from build123d import *

# Parameters (mm, degrees)
ESBO_O1_R                = 1.25
ESBO_O1_R_2              = 0.5
RESSALTO_EXTRUS_O1_DEPTH = 2
ESBO_O2_R                = 3.25
ESBO_O2_R_2              = 2.1
RESSALTO_EXTRUS_O2_DEPTH = 2.2


with BuildPart() as part:
    # Esboço1 → Ressalto-extrusão1 (new body)
    with BuildSketch(Plane.XY):
        with BuildLine():
            Line((16.1640625, 1.742292598), (0.3046875, 3.235686253))
            ThreePointArc((0.3046875, 3.235686253), (-3.25, 0), (0.3046875, -3.235686253))
            Line((0.3046875, -3.235686253), (16.1640625, -1.742292598))
            ThreePointArc((16.1640625, -1.742292598), (17.75, 0), (16.1640625, 1.742292598))
        make_face()
        Circle(ESBO_O1_R, mode=Mode.SUBTRACT)
        with Locations((16, 0)):
            Circle(ESBO_O1_R_2, mode=Mode.SUBTRACT)
        with Locations((14.03, 0)):
            Circle(ESBO_O1_R_2, mode=Mode.SUBTRACT)
        with Locations((12.06, 0)):
            Circle(ESBO_O1_R_2, mode=Mode.SUBTRACT)
        with Locations((10.09, 0)):
            Circle(ESBO_O1_R_2, mode=Mode.SUBTRACT)
        with Locations((8.12, 0)):
            Circle(ESBO_O1_R_2, mode=Mode.SUBTRACT)
        with Locations((6.15, 0)):
            Circle(ESBO_O1_R_2, mode=Mode.SUBTRACT)
        with Locations((4.18, 0)):
            Circle(ESBO_O1_R_2, mode=Mode.SUBTRACT)
    extrude(amount=RESSALTO_EXTRUS_O1_DEPTH)

    # Esboço2 → Ressalto-extrusão2 (add)
    with BuildSketch(Plane.XY.offset(2)):
        with Locations(Location((0, 0, 0), (0, 0, 275.379378991))):
            Circle(ESBO_O2_R)
        Circle(ESBO_O2_R_2, mode=Mode.SUBTRACT)
    extrude(amount=RESSALTO_EXTRUS_O2_DEPTH)


solid = part.part
CAD build for the part. Positions are in the model's coordinates, mm. A direction names the side the tool comes from. Coordinates: 2 decimals unless noted, no trailing zeros. Write each loop counter-clockwise with the first axis right and the second up, starting at its lowest first coordinate (ties: lowest second). Pieces come first, ordered by that corner, then holes. Notation, with made-up numbers: M 11.5,25.5 L 70.5,25.5 A33 cw 70.5,64.5 Z; hole C 55.5,18 d8. An arc over 180 degrees is marked long. Answer as a JSON object with one key per item and string values. Group by question number.
1) Saw through at B-B (z = 0.3). Give the number of separate pieces and of enclosed holes in the cut face, plus the area to 3 significant figures.
2) Tool access for faces 1 (the face through (1, -1, 2)), 2 (the face through (8.35, 2.48, 0.99)): list every direction of +Z, -Z, +X, -X, +Y, -Y with a clear straight run to the whole face (end or side of a thin tool).
3) Saw through at D-D (x = 12.06). Write the cut outline in (y, z), plus the area to 4 significant figures.
4) Pin check, flat tips, straight feed: pin 1 Ø1.5 at (x, z) = (11.5, 1.5) entering from +Y; pin 2 Ø3 at (x, y) = (8.5, 0) entering from +Z; pin 3 Ø2 at (x, z) = (9.5, 3.5) entering from -Y. Stop position of each tip, or through.
5) Saw through at C-C (y = 2.5). Write the cut outline in (x, z).
6) Mould opens along X. For faces 3 (the face through (7, 0, 0)), 4 (the face through (8.1, -2.5, 1)), 5 (the face through (2.003, 0.631, 3.085)) say: +X half, -X half, draft (parallel to the pull), parting line (faces both ways), or undercut.
7) Saw through at A-A (x = 0). Write the cut outline in (y, z).
8) Wall check: line 1 (Y direction, x = 0, z = 2.6); line 2 (Z direction, x = 5, y = -1); line 3 (X direction, y = 0.25, z = 3.75). Give the ranges that are in metal, low to high. Write a range as from..to.
Values follow:
{
 "1": {"separate pieces": "1", "enclosed holes": "8", "area": "91.3 mm2"},
 "2": {"face 1": "+Z", "face 2": "+Z, -Z, +X, +Y"},
 "3": {"outline": "M -2.13,0 L -0.5,0 L -0.5,2 L -2.13,2 Z; M 0.5,0 L 2.13,0 L 2.13,2 L 0.5,2 Z", "area": "6.515 mm2"},
 "4": {"pin 1": "stops at y = 2.25", "pin 2": "stops at z = 2", "pin 3": "passes through"},
 "5": {"outline": "M -2.08,0 L 8.12,0 L 8.12,2 L 2.08,2 L 2.08,4.2 L -2.08,4.2 Z"},
 "6": {"face 3": "draft", "face 4": "+X half", "face 5": "undercut"},
 "7": {"outline": "M -3.25,0 L -1.25,0 L -1.25,2 L -2.1,2 L -2.1,4.2 L -3.25,4.2 Z; M 1.25,0 L 3.25,0 L 3.25,4.2 L 2.1,4.2 L 2.1,2 L 1.25,2 Z"},
 "8": {"line 1": "y = -3.25..-2.1, 2.1..3.25", "line 2": "z = 0..2", "line 3": "x = -3.24..-2.09, 2.09..3.24"}
}
